from build123d import *

# Parameters (mm, degrees)
SKETCH_1_W          = 8
SKETCH_1_H          = 8
EXTRUDE_1_DEPTH     = 38
SKETCH_3_R          = 1.6
CUT_EXTRUDE_1_DEPTH = 40.038442592
SKETCH_2_R          = 1.6
CUT_EXTRUDE_2_DEPTH = 40.038442592


with BuildPart() as part:
    # 草图1 → 凸台-拉伸1 (new body)
    with BuildSketch(Plane.XY):
        Rectangle(SKETCH_1_W, SKETCH_1_H)
    extrude(amount=EXTRUDE_1_DEPTH)

    # 草图3 → 切除-拉伸1 (cut, through all)
    with BuildSketch(Plane(origin=(0, 4, 0), x_dir=(1, 0, 0), z_dir=(0, 1, 0))):
        with Locations(Location((0, -13, 0), (0, 0, 270))):
            Circle(SKETCH_3_R)
        with Locations(Location((0, -25, 0), (0, 0, 90))):
            Circle(SKETCH_3_R)
    extrude(amount=-CUT_EXTRUDE_1_DEPTH, mode=Mode.SUBTRACT)

    # 草图2 → 切除-拉伸2 (cut, through all)
    with BuildSketch(Plane(origin=(4, 0, 0), x_dir=(0, 0, -1), z_dir=(1, 0, 0))):
        with Locations((-30, 0)):
            Circle(SKETCH_2_R)
        with Locations(Location((-8, 0, 0), (0, 0, 180))):
            Circle(SKETCH_2_R)
    extrude(amount=-CUT_EXTRUDE_2_DEPTH, mode=Mode.SUBTRACT)


solid = part.part
Could you check a few things on this model? Use its own coordinates, in mm. Round coordinates to 2 decimals unless told otherwise and drop trailing zeros. Loops run counter-clockwise (first coordinate to the right, second up) from the corner with the lowest first, then second, coordinate; pieces in that order, holes last. Notation, with made-up numbers: (-7.5, -11) -> (4.5, -11) arc R21 cw to (4.5, 4) -> close; hole circle Ø8 at (69.5, 20). An arc over 180 degrees is marked (long way). Use CSV: the item, a comma, the result in double quotes.
(1) Suppose I cut it at D-D on y = -2.5. Write out the boundary of the cut face in (x, z), plus the area to 3 significant figures.
Return value:
outline,"(-4, 0) -> (4, 0) -> (4, 38) -> (-4, 38) -> close; hole circle Ø3.2 at (0, 13); hole circle Ø3.2 at (0, 25)"
area,"288 mm²"
(2) If I drill on probe 1 along Y at (x, z) = (0.75, 30); probe 2 along Z at (x, y) = (-1, 1); probe 3 along Z at (x, y) = (-0.5, 2.25), over which ranges is the centre line in solid material (lowest first)? Write a range as [from, to].
Return value:
probe 1,"y = [-4, -1.6], [1.6, 4]"
probe 2,"z = [0, 6.75], [9.25, 11.75], [14.25, 23.75], [26.25, 28.75], [31.25, 38]"
probe 3,"z = [0, 11.48], [14.52, 23.48], [26.52, 38]"
(3) Suppose I cut it at B-B on y = -1. Write out the boundary of the cut face in (x, z), plus the area to 3 significant figures.
Return value:
outline,"(-4, 0) -> (4, 0) -> (4, 6.75) -> (-4, 6.75) -> close; (-4, 9.25) -> (4, 9.25) -> (4, 28.75) -> (-4, 28.75) -> close; (-4, 31.25) -> (4, 31.25) -> (4, 38) -> (-4, 38) -> close; hole circle Ø3.2 at (0, 13); hole circle Ø3.2 at (0, 25)"
area,"248 mm²"
(4) If we mould it in two halves opening along X, with no side actions, what happens to faces 1 (the cylindrical face through (0.07, 0.06, 11.4)), 2 (the flat face through (4, 0, 19)), 3 (the flat face through (0, 4, 19))? For each: +X half, -X half, draft (parallel to the pull), parting line (faces both ways), or undercut.
Return value:
face 1,"undercut"
face 2,"+X half"
face 3,"draft"
(5) Suppose I cut it at A-A on z = 13. Write out the boundary of the cut face in (x, y).
Return value:
outline,"(-4, -4) -> (-1.6, -4) -> (-1.6, 4) -> (-4, 4) -> close; (1.6, -4) -> (4, -4) -> (4, 4) -> (1.6, 4) -> close"
(6) Suppose I cut it at C-C on x = 0.5. Write out the boundary of the cut face in (y, z).
Return value:
outline,"(-4, 0) -> (4, 0) -> (4, 11.48) -> (-4, 11.48) -> close; (-4, 14.52) -> (4, 14.52) -> (4, 23.48) -> (-4, 23.48) -> close; (-4, 26.52) -> (4, 26.52) -> (4, 38) -> (-4, 38) -> close; hole circle Ø3.2 at (0, 8); hole circle Ø3.2 at (0, 30)"
